Could you check a few things on this drawing? It's one solid part, dimensions in mm from its lowest x, y, z. Give positions to 0.01 mm unless a question says otherwise; leave off trailing zeros. Loops run counter-clockwise (first coordinate to the right, second up) from the corner with the lowest first, then second, coordinate; pieces in that order, holes last. Notation, with made-up numbers: (-7, 52) -> (7, 52) arc R23 cw to (7, 84) -> close; hole circle Ø7 at (-28, 41). An arc over 180 degrees is marked (long way). One line per question, with ' | ' between items.
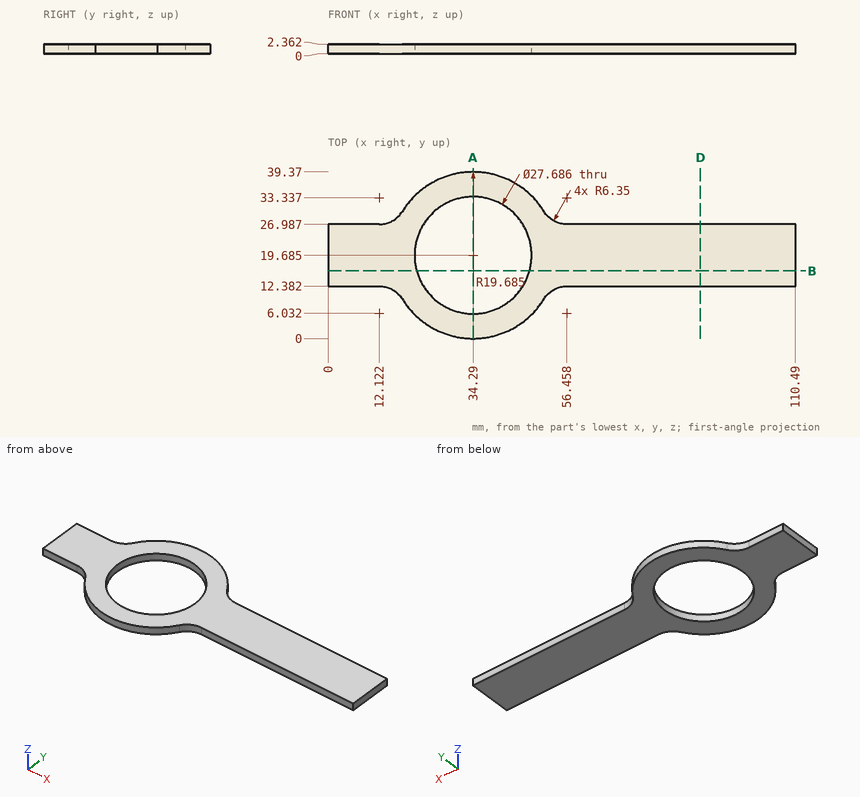
Q1. If we section it at D-D (x = 88): Write out the boundary of the cut face in (y, z).
Entries:
outline: (12.38, 0) -> (26.99, 0) -> (26.99, 2.36) -> (12.38, 2.36) -> close
Q2. For pin 1 Ø0.7 at (x, z) = (73.5, 1.5) entering from -Y; pin 2 Ø10 at (x, y) = (83.5, 30) entering from +Z, each with a flat end and sliding along its axis, tell me the tip position at first contact or that it passes through.
Entries:
pin 1: y = 12.38 | pin 2: z = 2.36
Q3. If we section it at B-B (y = 16): Write out the boundary of the cut face in (x, z), plus the area to 3 significant figures.
Entries:
outline: (0, 0) -> (20.95, 0) -> (20.95, 2.36) -> (0, 2.36) -> close; (47.63, 0) -> (110.49, 0) -> (110.49, 2.36) -> (47.63, 2.36) -> close | area: 198 mm²
Q4. If I drill on probe 1 along X at (y, z) = (21, 0.55); probe 2 along X at (y, z) = (29.5, 1.95); probe 3 along Y at (x, z) = (104, 1.25), over which ranges is the centre line in solid material (lowest first)? Write a range as from..to.
Entries:
probe 1: 0..20.51, 48.07..110.49 | probe 2: 17.18..24.53, 44.05..51.4 | probe 3: 12.38..26.99
Q5. If we section it at A-A (x = 34.29): Write out the boundary of the cut face in (y, z), plus the area to 3 significant figures.
Entries:
outline: (0, 0) -> (5.84, 0) -> (5.84, 2.36) -> (0, 2.36) -> close; (33.53, 0) -> (39.37, 0) -> (39.37, 2.36) -> (33.53, 2.36) -> close | area: 27.6 mm²
